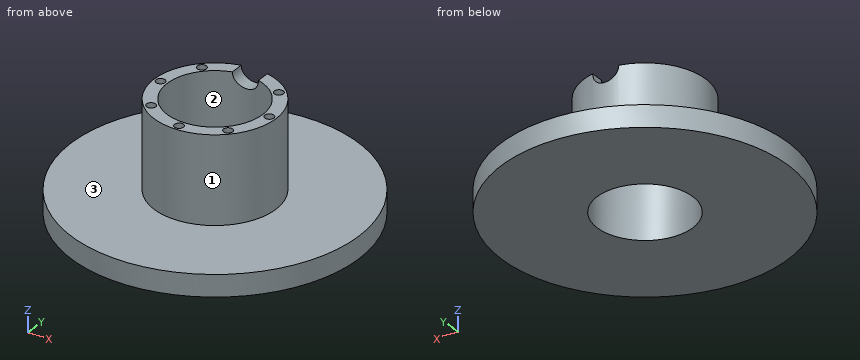
from build123d import *

# Parameters (mm, degrees)
F0_R     = 14
F0_R_2   = 11
F1_DEPTH = 25
F0_R_3   = 33
F2_DEPTH = 5
F3_R     = 3
F4_DEPTH = 25
F6_R     = 1.05
F7_DEPTH = 2


with BuildPart() as f1:
    # F0 (on Top) → F1 (new body)
    with BuildSketch(Plane.XY):
        Circle(F0_R)
        Circle(F0_R_2, mode=Mode.SUBTRACT)
    extrude(amount=F1_DEPTH)

    # F0 (on Top) → F2 (join)
    with BuildSketch(Plane.XY):
        Circle(F0_R_3)
        Circle(F0_R, mode=Mode.SUBTRACT)
    extrude(amount=F2_DEPTH)

    # F3 (on Front) → F4 (cut)
    with BuildSketch(Plane.XZ):
        with Locations((0, 25)):
            Circle(F3_R)
    extrude(amount=-F4_DEPTH, mode=Mode.SUBTRACT)

    # F6 (on offset) → F7 (cut)
    with BuildSketch(Plane.XY.offset(25)):
        with Locations((-8.8388347648, 8.8388347648)):
            Circle(F6_R)
        with Locations((8.8388347648, 8.8388347648)):
            Circle(F6_R)
        with Locations((12.5, 0)):
            Circle(F6_R)
        with Locations((8.8388347648, -8.8388347648)):
            Circle(F6_R)
        with Locations((0, -12.5)):
            Circle(F6_R)
        with Locations((-8.8388347648, -8.8388347648)):
            Circle(F6_R)
        with Locations((-12.5, 0)):
            Circle(F6_R)
    extrude(amount=-F7_DEPTH, mode=Mode.SUBTRACT)


solid = f1.part
Read the model definition and answer for the solid it produces. Units are mm, in the model's axes. Face numbers are marked on the shaded views. Coordinates: 2 decimals unless noted, no trailing zeros. Loops run counter-clockwise (first coordinate to the right, second up) from the corner with the lowest first, then second, coordinate; pieces in that order, holes last. Notation, with made-up numbers: (18.25, 81.25) -> (53.25, 81.25) arc R25 cw to (53.25, 113.25) -> close; hole circle Ø10 at (-37, 59.5). An arc over 180 degrees is marked (long way). Write item = value, one per line. Start each with the question number.
1) The part is cut by section D-D, the plane z = 14. Determine the outline of the cut face in (x, y).
2) The part is cut by section B-B, the plane z = 3.5. Determine the outline of the cut face in (x, y).
3) The mould has two halves that part along Y. Classify the marked faces 1, 2 and 3: pulls with the +Y half, pulls with the -Y half, needs draft (parallel to the pull), parting line crosses it, or undercut.
4) The part is cut by section C-C, the plane x = 12.5. Determine the outline of the cut face in (y, z).
5) The part is cut by section A-A, the plane y = 0. Determine the outline of the cut face in (x, z), plus the area to 3 significant figures.
6) Given P1, Ø4, axis at y = -16, z = 4, coming from the +X side; P2, Ø8, axis at x = 15.5, z = 17.5, coming from the -Y side; P3, Ø1, axis at x = 12, y = 0, coming from the +Z side; P4, Ø20, axis at x = 0, y = 0, coming from the -Z side, each flat-ended and moving along its own axis, determine where each tip first touches the part or whether it passes through.
7) Find the intervals of material crossed by L1, parallel to Y at x = 0, z = 15.5; L2, parallel to Y at x = 0, z = 24.1; L3, parallel to Z at x = 19, y = -10.5, in increasing order. Write a range as from..to.
Result:
q1.outline = circle Ø28 at (0, 0); hole circle Ø22 at (0, 0)
q2.outline = circle Ø66 at (0, 0); hole circle Ø22 at (0, 0)
q3.face_1 = parting line crosses it
q3.face_2 = undercut
q3.face_3 = needs draft
q4.outline = (-30.54, 0) -> (30.54, 0) -> (30.54, 5) -> (6.3, 5) -> (6.3, 25) -> (1.05, 25) -> (1.05, 23) -> (-1.05, 23) -> (-1.05, 25) -> (-6.3, 25) -> (-6.3, 5) -> (-30.54, 5) -> close
q5.outline = (-33, 0) -> (-11, 0) -> (-11, 25) -> (-11.45, 25) -> (-11.45, 23) -> (-13.55, 23) -> (-13.55, 25) -> (-14, 25) -> (-14, 5) -> (-33, 5) -> close; (11, 0) -> (33, 0) -> (33, 5) -> (14, 5) -> (14, 25) -> (13.55, 25) -> (13.55, 23) -> (11.45, 23) -> (11.45, 25) -> (11, 25) -> close
q5.area = 332 mm²
q6.P1 = 29.88
q6.P2 = -7.98
q6.P3 = 23
q6.P4 = through
q7.L1 = -14..-11, 11..14
q7.L2 = -14..-13.55, -11.45..-11
q7.L3 = 0..5
